Build history of the part. All positions in model axes, mm. A direction names the side the tool comes from. Round coordinates to 2 decimals unless told otherwise and drop trailing zeros. Loops run counter-clockwise (first coordinate to the right, second up) from the corner with the lowest first, then second, coordinate; pieces in that order, holes last. Notation, with made-up numbers: (-9.75, -22) -> (-3.75, -22) arc R23 ccw to (-3.75, -9) -> close; hole circle Ø10 at (-8, 12.25). An arc over 180 degrees is marked (long way). Put each result on its own line as item: value. Start each with the question number.
Item 1: Tool access for faces 4 (the flat face through (32.39, 17.54, 46.36)), 5 (the flat face through (4, 40, 20)), 6 (the flat face through (46.394, 27.63, 17.535)), 7 (the flat face through (17.54, 42.61, 28.64)): list every direction of +Z, -Z, +X, -X, +Y, -Y with a clear straight run to the whole face (end or side of a thin tool).
Item 2: Drill centre lines: probe 1 along Z at (x, y) = (30, 10); probe 2 along X at (y, z) = (29.5, 12); probe 3 along Y at (x, z) = (39, 10). Where is each one in solid material? Low to high. Write a range as [from, to].
Item 3: Pull direction Y, two halves, no side cores. Call faces 1 (the flat face through (20, 0, 14)), 2 (the flat face through (39, 39, 8)), 3 (the flat face through (46.3, 28.6, 15)): +Y half, -Y half, draft (parallel to the pull), parting line (faces both ways), or undercut.
Item 4: Cut at C-C, the plane y = 10. List the corners of the cut face in (x, z).
Item 5: Cut at A-A, the plane y = 45. Count the separate pieces of the cut face and the enclosed holes in it, plus the area to 3 significant figures.
Item 6: Flat gauge pins, fed straight in: pin 1 Ø5.5 at (y, z) = (3.5, 44.5) entering from +X; pin 2 Ø5.5 at (x, y) = (45, 30) entering from -Z; pin 3 Ø2 at (x, z) = (52.5, 49) entering from -Y; pin 4 Ø8 at (x, y) = (10.5, 10.5) entering from +Z. Where does each tip first touch, or does it go through?
Item 7: Cut at B-B, the plane z = 53. List the corners of the cut face in (x, y), plus the area to 3 significant figures.
```python
from build123d import *

# Parameters (mm, degrees)
BASE_SHAPE_BASE_DEPTH        = 20
BASE_SHAPE_EXTENSION_DEPTH   = 40
BASE_SHAPE_FINISH_SKETCH_W   = 12
BASE_SHAPE_FINISH_SKETCH_H   = 40
BASE_SHAPE_WALL_DEPTH        = 40
ROD_HOLE_D10_Z_D             = 10.2
ROD_HOLE_D10_Z_DEPTH         = 40
ROD_HOLE_D10_Z_CSINK_D       = 10.5
ROD_HOLE_D10_Z_CSINK_ANGLE   = 60
ROD_HOLE_D10_X_D             = 10.2
ROD_HOLE_D10_X_DEPTH         = 40
ROD_HOLE_D10_X_CSINK_D       = 10.5
ROD_HOLE_D10_X_CSINK_ANGLE   = 60
ROD_HOLE_D10_Y_D             = 10.2
ROD_HOLE_D10_Y_DEPTH         = 40
ROD_HOLE_D10_Y_CSINK_D       = 10.5
ROD_HOLE_D10_Y_CSINK_ANGLE   = 60
OUTER_CHAMFERS_SIZE          = 5
INNER_SMALLER_CHAMFERS_SIZE  = 1
LARGE_CHAMFERS_SIZE          = 20
HULL_PART_HOLES_M3_START     = 8
HULL_PART_HOLES_M3_OUTLINE_R = 1.7
HULL_PART_HOLES_M3_DEPTH     = 12
HULL_PART_NUT_HOLE_DEPTH     = 5


# Read off the part's stored shape, not the designer's step: hull_part_holes_m3
with BuildPart() as part:
    # base_shape_sketch → base_shape_base (new body)
    with BuildSketch(Plane.XY):
        Polygon((0, 0), (60, 0), (60, 20), (20, 20), (20, 60), (0, 60), align=None)
    extrude(amount=BASE_SHAPE_BASE_DEPTH)

    # base_shape_extension_sketch → base_shape_extension (add)
    with BuildSketch(Plane.XY.offset(20)):
        Polygon((20, 60), (20, 20), (60, 20), (60, 8), (20, 8), (20, 0), (0, 0), (0, 20), (8, 20), (8, 60), align=None)
    extrude(amount=BASE_SHAPE_EXTENSION_DEPTH)

    # base_shape_finish_sketch → base_shape_wall (add)
    with BuildSketch(Plane(origin=(20, 0, 0), x_dir=(0, 0, -1), z_dir=(1, 0, 0))):
        with Locations((-14, 40)):
            Rectangle(BASE_SHAPE_FINISH_SKETCH_W, BASE_SHAPE_FINISH_SKETCH_H)
    extrude(amount=BASE_SHAPE_WALL_DEPTH)

    # rod_hole_d10_z
    with Locations(Plane.XY.offset(60)):
        with Locations((10, 10)):
            CounterSinkHole(ROD_HOLE_D10_Z_D / 2, ROD_HOLE_D10_Z_CSINK_D / 2, depth=ROD_HOLE_D10_Z_DEPTH, counter_sink_angle=ROD_HOLE_D10_Z_CSINK_ANGLE)

    # rod_hole_d10_x
    with Locations(Plane(origin=(60, 0, 0), x_dir=(0, 0, -1), z_dir=(1, 0, 0))):
        with Locations((-10, 10)):
            CounterSinkHole(ROD_HOLE_D10_X_D / 2, ROD_HOLE_D10_X_CSINK_D / 2, depth=ROD_HOLE_D10_X_DEPTH, counter_sink_angle=ROD_HOLE_D10_X_CSINK_ANGLE)

    # rod_hole_d10_y
    with Locations(Plane(origin=(0, 60, 0), x_dir=(1, 0, 0), z_dir=(0, 1, 0))):
        with Locations((10, -10)):
            CounterSinkHole(ROD_HOLE_D10_Y_D / 2, ROD_HOLE_D10_Y_CSINK_D / 2, depth=ROD_HOLE_D10_Y_DEPTH, counter_sink_angle=ROD_HOLE_D10_Y_CSINK_ANGLE)

    # outer_chamfers
    outer_chamfers_edges = [part.edges().sort_by_distance(p)[0] for p in [
        (0, 0, 30),
        (30, 0, 0),
        (0, 30, 0),
    ]]
    chamfer(outer_chamfers_edges, length=OUTER_CHAMFERS_SIZE)

    # inner_smaller_chamfers
    inner_smaller_chamfers_edges = [part.edges().sort_by_distance(p)[0] for p in [
        (0, 60, 12.5),
        (60, 0, 12.5),
        (60, 4, 20),
        (40, 0, 20),
        (4, 60, 20),
        (0, 20, 40),
        (20, 0, 40),
        (4, 20, 60),
        (0, 12.5, 60),
        (20, 4, 60),
        (20, 60, 4),
        (0, 40, 20),
        (60, 20, 4),
        (12.5, 60, 0),
        (20, 40, 0),
        (40, 20, 0),
        (12.5, 0, 60),
        (2.5, 2.5, 60),
        (60, 12.5, 0),
        (60, 2.5, 2.5),
        (2.5, 60, 2.5),
    ]]
    chamfer(inner_smaller_chamfers_edges, length=INNER_SMALLER_CHAMFERS_SIZE)

    # large_chamfers
    large_chamfers_edges = [part.edges().sort_by_distance(p)[0] for p in [
        (14, 60, 60),
        (60, 14, 60),
        (60, 60, 14),
    ]]
    chamfer(large_chamfers_edges, length=LARGE_CHAMFERS_SIZE)

    # hull_part_holes_m3 outline → hull_part_holes_m3 (cut)
    with BuildSketch(Plane.YZ.offset(HULL_PART_HOLES_M3_START)):
        with Locations((45, 30)):
            Circle(HULL_PART_HOLES_M3_OUTLINE_R)
        with Locations((30, 45)):
            Circle(HULL_PART_HOLES_M3_OUTLINE_R)
    hull_part_holes_m3 = extrude(amount=HULL_PART_HOLES_M3_DEPTH, mode=Mode.SUBTRACT)

    # Sketch12 → hull_part_nut_hole (cut)
    with BuildSketch(Plane(origin=(20, 0, 0), x_dir=(0, 0, -1), z_dir=(1, 0, 0))):
        Polygon((-30, 48.175426481), (-32.75, 46.58771324), (-32.75, 43.41228676), (-30, 41.824573519), (-27.25, 43.41228676), (-27.25, 46.58771324), align=None)
        Polygon((-45, 33.175426481), (-47.75, 31.58771324), (-47.75, 28.41228676), (-45, 26.824573519), (-42.25, 28.41228676), (-42.25, 31.58771324), align=None)
    hull_part_nut_hole = extrude(amount=-HULL_PART_NUT_HOLE_DEPTH, mode=Mode.SUBTRACT)

    # hull_part_holes_mirror_x: hull_part_holes_m3, hull_part_nut_hole across plane
    add(hull_part_holes_m3.mirror(Plane(origin=(0, 0, 0), x_dir=(0.7071067811865482, 0, 0.7071067811865468), z_dir=(-0.707106781186547, 0, 0.7071067811865481))), mode=Mode.SUBTRACT)
    add(hull_part_nut_hole.mirror(Plane(origin=(0, 0, 0), x_dir=(0.7071067811865482, 0, 0.7071067811865468), z_dir=(-0.707106781186547, 0, 0.7071067811865481))), mode=Mode.SUBTRACT)

    # hull_part_holes_mirror_y: hull_part_holes_m3, hull_part_nut_hole across plane
    add(hull_part_holes_m3.mirror(Plane(origin=(0, 0, 0), x_dir=(0, 0, 1), z_dir=(-0.7071067811865482, 0.7071067811865469, 0))), mode=Mode.SUBTRACT)
    add(hull_part_nut_hole.mirror(Plane(origin=(0, 0, 0), x_dir=(0, 0, 1), z_dir=(-0.7071067811865482, 0.7071067811865469, 0))), mode=Mode.SUBTRACT)


solid = part.part
```
Reply:
1. face 4: +Y
1. face 5: +Z, -X, +Y
1. face 6: +Z
1. face 7: +X
2. probe 1: z = [0, 4.9], [15.1, 43.3], [46.7, 60]
2. probe 2: x = [0, 5.31], [14.69, 43.38], [46.62, 60]
2. probe 3: y = [0, 4.9], [15.1, 60]
3. face 1: -Y half
3. face 2: draft
3. face 3: undercut
4. outline: (0, 5) -> (5, 0) -> (59, 0) -> (60, 1) -> (60, 4.75) -> (59.74, 4.9) -> (20, 4.9) -> (20, 15.1) -> (59.74, 15.1) -> (60, 15.25) -> (60, 40) -> (40, 60) -> (15.25, 60) -> (15.1, 59.74) -> (15.1, 20) -> (4.9, 20) -> (4.9, 59.74) -> (4.75, 60) -> (1, 60) -> (0, 59) -> close; hole circle Ø3.4 at (30, 45); hole circle Ø3.4 at (45, 30)
5. separate pieces: 3
5. enclosed holes: 1
5. area: 1,040 mm^2
6. pin 1: stops at x = 20
6. pin 2: stops at z = 8
6. pin 3: passes through
6. pin 4: stops at z = 20
7. outline: (0, 5) -> (5, 0) -> (19, 0) -> (20, 1) -> (20, 8) -> (47, 8) -> (47, 20) -> (20, 20) -> (20, 47) -> (8, 47) -> (8, 20) -> (1, 20) -> (0, 19) -> close; hole circle Ø10.2 at (10, 10)
7. area: 953 mm^2
